Model file for the job. Use its own axes, mm. A direction names the side the tool comes from. Coordinates: 2 decimals unless noted, no trailing zeros. Order: outer loops, then holes, each group sorted by start corner. A loop starts at its lowest first (then second) coordinate and runs counter-clockwise, first axis right, second up. Notation, with made-up numbers: (-8, 37.5) -> (25, 37.5) arc R22 ccw to (25, 43.5) -> close; hole circle Ø11 at (36, -22.75). An arc over 180 degrees is marked (long way). Use CSV: the item, a comma, the result in double quotes. Start each with the question number.
(1) Pull direction X, two halves, no side cores. Call faces 1 (the flat face through (2.79, -1.09, 1.39)), 2 (the flat face through (0.94, 0, 5)), 3 (the cylindrical face through (2.192, -4.214, 14.79)): pulls with the +X half, pulls with the -X half, needs draft (parallel to the pull), parting line crosses it, or undercut.
(2) Pin check, flat tips, straight feed: pin 1 Ø1.5 at (y, z) = (1.5, 5) entering from +X; pin 2 Ø3 at (y, z) = (-2, 5.5) entering from -X; pin 3 Ø1.4 at (x, y) = (-0.5, 0) entering from -Z. Stop position of each tip, or through.
(3) Tool access for faces 4 (the flat face through (0, 0, 30)), 5 (the flat face through (2.79, 1.09, 2.61)), 6 (the flat face through (0, 0, 10)): list every direction of +Z, -Z, +X, -X, +Y, -Y with a clear straight run to the whole face (end or side of a thin tool).
(4) Probe L1, parallel to Y at x = 0, z = 7.5; L2, parallel to X at y = 0.25, z = 10.25; L3, parallel to Z at x = 3.5, y = 0.5. List the from-to ranges inside material, lowest first.
(5) Cut at B-B on x = 1.25. Write the cut outline in (y, z).
(6) Cut at D-D on z = 20. Write the cut outline in (x, y).
(7) Cut at A-A on y = 0. Write the cut outline in (x, z).
(8) Cut at C-C on x = 0. Write the cut outline in (y, z).
```python
from build123d import *

# Parameters (mm, degrees)
SKETCH1_R           = 4.75
BOSS_EXTRUDE1_DEPTH = 30
CUT_EXTRUDE1_DEPTH  = 10
CUT_EXTRUDE2_DEPTH  = 31.902080836


with BuildPart() as part:
    # Sketch1 → Boss-Extrude1 (new body)
    with BuildSketch(Plane.XY):
        Circle(SKETCH1_R)
    extrude(amount=BOSS_EXTRUDE1_DEPTH)

    # Sketch2 → Cut-Extrude1 (cut)
    with BuildSketch(Plane(origin=(0, 0, 0), x_dir=(-1, 0, 0), z_dir=(0, 0, -1))):
        with BuildLine():
            Line((-0.94, 1.535057002), (-0.94, -1.535057002))
            ThreePointArc((-0.94, -1.535057002), (1.8, 0), (-0.94, 1.535057002))
        make_face()
    extrude(amount=-CUT_EXTRUDE1_DEPTH, mode=Mode.SUBTRACT)

    # Sketch3 → Cut-Extrude2 (cut, through all)
    with BuildSketch(Plane.ZY.offset(-0.94)):
        Polygon((3.230708553, 0.754115238), (1.962271323, 1.44288249), (0.73156277, 0.688767252), (0.769291447, -0.754115238), (2.037728677, -1.44288249), (3.26843723, -0.688767252), align=None)
    extrude(amount=-CUT_EXTRUDE2_DEPTH, mode=Mode.SUBTRACT)


solid = part.part
```
Outcome:
1,face 1,"needs draft"
1,face 2,"undercut"
1,face 3,"parting line crosses it"
2,pin 1,"x = 4.69"
2,pin 2,"x = -4.72"
2,pin 3,"z = 10"
3,face 4,"+Z, +X, -X, +Y, -Y"
3,face 5,"+X"
3,face 6,"-Z"
4,L1,"-4.75 to -1.8, 1.8 to 4.75"
4,L2,"-4.74 to 4.74"
4,L3,"0 to 0.74, 3.24 to 30"
5,outline,"(-4.58, 0) -> (4.58, 0) -> (4.58, 30) -> (-4.58, 30) -> close; hole (-1.44, 2.04) -> (-0.75, 0.77) -> (0.69, 0.73) -> (1.44, 1.96) -> (0.75, 3.23) -> (-0.69, 3.27) -> close"
6,outline,"circle Ø9.5 at (0, 0)"
7,outline,"(-4.75, 0) -> (-1.8, 0) -> (-1.8, 10) -> (0.94, 10) -> (0.94, 3.25) -> (4.75, 3.25) -> (4.75, 30) -> (-4.75, 30) -> close; (0.94, 0) -> (4.75, 0) -> (4.75, 0.75) -> (0.94, 0.75) -> close"
8,outline,"(-4.75, 0) -> (-1.8, 0) -> (-1.8, 10) -> (1.8, 10) -> (1.8, 0) -> (4.75, 0) -> (4.75, 30) -> (-4.75, 30) -> close"
